Check sheet for the modelled part. Datum: model origin and axes. Units: mm. A direction names the side the tool comes from. Coordinates: 2 decimals unless noted, no trailing zeros. Write each loop counter-clockwise with the first axis right and the second up, starting at its lowest first coordinate (ties: lowest second). Pieces come first, ordered by that corner, then holes. Notation, with made-up numbers: (-23, 32.25) -> (19, 32.25) arc R9 ccw to (19, 48.25) -> close; hole circle Ø8 at (22.5, 17). An arc over 180 degrees is marked (long way). One line per item, written item: value. Start each with the question number.
1) Sectioned sample at A-A on y = 12. Enter the section's corners in (x, z).
2) Set-up check for faces 1 (the flat face through (20.549, 5.535, 27.849)), 2 (the cylindrical face through (23.89, 1.52, 47.74)), 3 (the flat face through (21, 42, 43)): record each of +Z, -Z, +X, -X, +Y, -Y from which the full face is reachable in a straight line by a thin tool's end or side.
3) Sectioned sample at B-B on z = -0.5. Enter the section's corners in (x, y).
4) Sectioned sample at D-D on x = 7. Enter the section's corners in (y, z), plus the area to 3 significant figures.
5) Gauge pin test, flat ends, axial feed: P1, Ø3.5, axis at y = 43.5, z = 44, coming from the -X side; P2, Ø5, axis at x = -1.96, z = -5.14, coming from the -Y side; P3, Ø6, axis at y = 7.5, z = 2.5, coming from the -X side; P4, Ø1.8, axis at y = 42.5, z = 48.61, coming from the +X side. Record the tip position at first contact, or that the pin passes through.
6) Sectioned sample at C-C on z = 36. Enter the section's corners in (x, y), plus the area to 3 significant figures.
7) Draft check along Y on faces 4 (the cylindrical face through (17.9, 1.5, 40.9)), 5 (the flat face through (18, 19, 40.314)), 6 (the flat face through (25, 44.5, 36)). Enter one of: +Y half, -Y half, draft (parallel to the pull), parting line (faces both ways), or undercut.
8) Scan lines: line 1 along Z through (x, y) = (19.5, 31); line 2 along Y through (x, z) = (6, 15); line 3 along X through (y, z) = (42, 31). Record each from-to range of solid material in increasing order. Write a range as [from, to].
```python
from build123d import *

# Parameters (mm, degrees)
SKETCH1_R           = 1.6
BOSS_EXTRUDE1_DEPTH = 3
SKETCH2_W           = 10
SKETCH2_H           = 10
BOSS_EXTRUDE2_DEPTH = 42
CHAMFER1_SIZE       = 5
SKETCH3_R           = 2.1
CUT_EXTRUDE1_DEPTH  = 52
SKETCH4_R           = 2.65
CUT_EXTRUDE2_DEPTH  = 0.5
SKETCH11_W          = 6
SKETCH11_H          = 3
BOSS_EXTRUDE7_DEPTH = 8
SKETCH12_R          = 1.2
CUT_EXTRUDE5_DEPTH  = 72.139584736
FILLET1_R           = 2
SKETCH13_W          = 2
SKETCH13_H          = 3
BOSS_EXTRUDE8_DEPTH = 10
SKETCH14_W          = 2
SKETCH14_H          = 10
BOSS_EXTRUDE9_DEPTH = 3
SKETCH15_R          = 1.5
CUT_EXTRUDE6_DEPTH  = 3


with BuildPart() as part:
    # Sketch1 → Boss-Extrude1 (new body)
    with BuildSketch(Plane(origin=(0, 0, 0), x_dir=(1, 0, 0), z_dir=(0, 1, 0))):
        Polygon((-6.512396694, 9.685950413), (1.487603306, 9.685950413), (26.487603306, 9.685950413), (26.487603306, -40.314049587), (1.487603306, -40.314049587), (-6.512396694, -40.314049587), align=None)
        with Locations(Location((-1.962396694, -35.764049587, 0), (0, 0, 270))):
            Circle(SKETCH1_R, mode=Mode.SUBTRACT)
        with Locations(Location((-1.962396694, 5.135950413, 0), (0, 0, 270))):
            Circle(SKETCH1_R, mode=Mode.SUBTRACT)
    extrude(amount=BOSS_EXTRUDE1_DEPTH)

    # Sketch2 → Boss-Extrude2 (add)
    with BuildSketch(Plane(origin=(0, 3, 0), x_dir=(1, 0, 0), z_dir=(0, 1, 0))):
        with Locations((21.487603306, -35.314049587)):
            Rectangle(SKETCH2_W, SKETCH2_H)
        with Locations((21.487603306, 4.685950413)):
            Rectangle(SKETCH2_W, SKETCH2_H)
    extrude(amount=BOSS_EXTRUDE2_DEPTH)

    # Chamfer1
    chamfer1_edges = [part.edges().sort_by_distance(p)[0] for p in [
        (21.487603306, 3, 30.314049587),
        (16.487603306, 3, 35.314049587),
        (16.487603306, 3, -4.685950413),
        (21.487603306, 3, 0.314049587),
    ]]
    chamfer(chamfer1_edges, length=CHAMFER1_SIZE)

    # Sketch3 → Cut-Extrude1 (cut)
    with BuildSketch(Plane(origin=(0, 45, 0), x_dir=(1, 0, 0), z_dir=(0, 1, 0))):
        with Locations(Location((22.537603306, -36.364049587, 0), (0, 0, 270))):
            Circle(SKETCH3_R)
        with Locations(Location((22.537603306, 5.735950413, 0), (0, 0, 270))):
            Circle(SKETCH3_R)
    extrude(amount=-CUT_EXTRUDE1_DEPTH, mode=Mode.SUBTRACT)

    # Sketch4 → Cut-Extrude2 (cut)
    with BuildSketch(Plane(origin=(0, 45, 0), x_dir=(1, 0, 0), z_dir=(0, 1, 0))):
        with Locations(Location((22.537603306, -36.364049587, 0), (0, 0, 270))):
            Circle(SKETCH4_R)
        with Locations(Location((22.537603306, 5.735950413, 0), (0, 0, 270))):
            Circle(SKETCH4_R)
    cut_extrude2 = extrude(amount=-CUT_EXTRUDE2_DEPTH, mode=Mode.SUBTRACT)

    # Mirror1: Cut-Extrude2 across plane
    add(cut_extrude2.mirror(Plane(origin=(0, 22.5, 0), x_dir=(0, 0, 1), z_dir=(0, -1, 0))), mode=Mode.SUBTRACT)

    # Sketch11 → Boss-Extrude7 (add)
    with BuildSketch(Plane.XY.offset(40.314049587)):
        with Locations((21.487603306, 43.5)):
            Rectangle(SKETCH11_W, SKETCH11_H)
        with Locations((21.487603306, 1.5)):
            Rectangle(SKETCH11_W, SKETCH11_H)
    extrude(amount=BOSS_EXTRUDE7_DEPTH)

    # Sketch12 → Cut-Extrude5 (cut, through all)
    with BuildSketch(Plane.XZ):
        with Locations(Location((21.487603306, 45.314049587, 0), (0, 0, 270))):
            Circle(SKETCH12_R)
    extrude(amount=-CUT_EXTRUDE5_DEPTH, mode=Mode.SUBTRACT)

    # Fillet1
    fillet1_edges = [part.edges().sort_by_distance(p)[0] for p in [
        (18.487603306, 43.5, 40.314049587),
        (18.487603306, 1.5, 40.314049587),
        (24.487603306, 1.5, 40.314049587),
    ]]
    fillet(fillet1_edges, radius=FILLET1_R - 0.0001)  # a hair under: the kernel refuses the full size
    fillet1_2_edges = [part.edges().sort_by_distance(p)[0] for p in [
        (18.487603306, 43.5, 48.314049587),
        (24.487603306, 1.5, 48.314049587),
        (18.487603306, 1.5, 48.314049587),
    ]]
    fillet(fillet1_2_edges, radius=FILLET1_R)

    # Sketch13 → Boss-Extrude8 (add)
    with BuildSketch(Plane.XY.offset(40.314049587)):
        with Locations((25.487603306, 43.5)):
            Rectangle(SKETCH13_W, SKETCH13_H)
    extrude(amount=BOSS_EXTRUDE8_DEPTH)

    # Sketch14 → Boss-Extrude9 (add)
    with BuildSketch(Plane.XZ.offset(-42)):
        with Locations((25.487603306, 45.314049587)):
            Rectangle(SKETCH14_W, SKETCH14_H)
    extrude(amount=BOSS_EXTRUDE9_DEPTH)

    # Sketch15 → Cut-Extrude6 (cut)
    with BuildSketch(Plane(origin=(26.487603306, 0, 0), x_dir=(0, 0, -1), z_dir=(1, 0, 0))):
        with Locations((-48.614049587, 42.5)):
            Circle(SKETCH15_R)
    extrude(amount=-CUT_EXTRUDE6_DEPTH, mode=Mode.SUBTRACT)


solid = part.part
```
Answers:
1. outline: (16.49, -9.69) -> (26.49, -9.69) -> (26.49, 0.31) -> (16.49, 0.31) -> close; (16.49, 30.31) -> (26.49, 30.31) -> (26.49, 40.31) -> (16.49, 40.31) -> close; hole circle Ø4.2 at (22.54, -5.74); hole circle Ø4.2 at (22.54, 36.36)
2. face 1: +X, -X, +Y
2. face 2: +Z, +X, -Y
2. face 3: +Z, -X
3. outline: (-6.51, 0) -> (26.49, 0) -> (26.49, 45) -> (16.49, 45) -> (16.49, 8) -> (11.49, 3) -> (-6.51, 3) -> close
4. outline: (0, -9.69) -> (3, -9.69) -> (3, 40.31) -> (0, 40.31) -> close
4. area: 150 mm2
5. P1: stops at x = 18.49
5. P2: stops at y = 0
5. P3: stops at x = 12.99
5. P4: stops at x = 23.49
6. outline: (-6.51, 0) -> (-3.54, 0) -> (-3.54, 3) -> (-6.51, 3) -> close; (-0.38, 0) -> (19.91, 0) -> (19.91, 0.5) -> (20.47, 0.5) -> (20.47, 44.5) -> (19.91, 44.5) -> (19.91, 45) -> (16.49, 45) -> (16.49, 8) -> (11.49, 3) -> (-0.38, 3) -> close; (24.61, 0.5) -> (25.16, 0.5) -> (25.16, 0) -> (26.49, 0) -> (26.49, 45) -> (25.16, 45) -> (25.16, 44.5) -> (24.61, 44.5) -> close
6. area: 335 mm2
7. face 4: draft
7. face 5: undercut
7. face 6: +Y half
8. line 1: z = [-9.69, 0.31], [30.31, 40.31]
8. line 2: y = [0, 3]
8. line 3: x = [16.49, 26.49]
